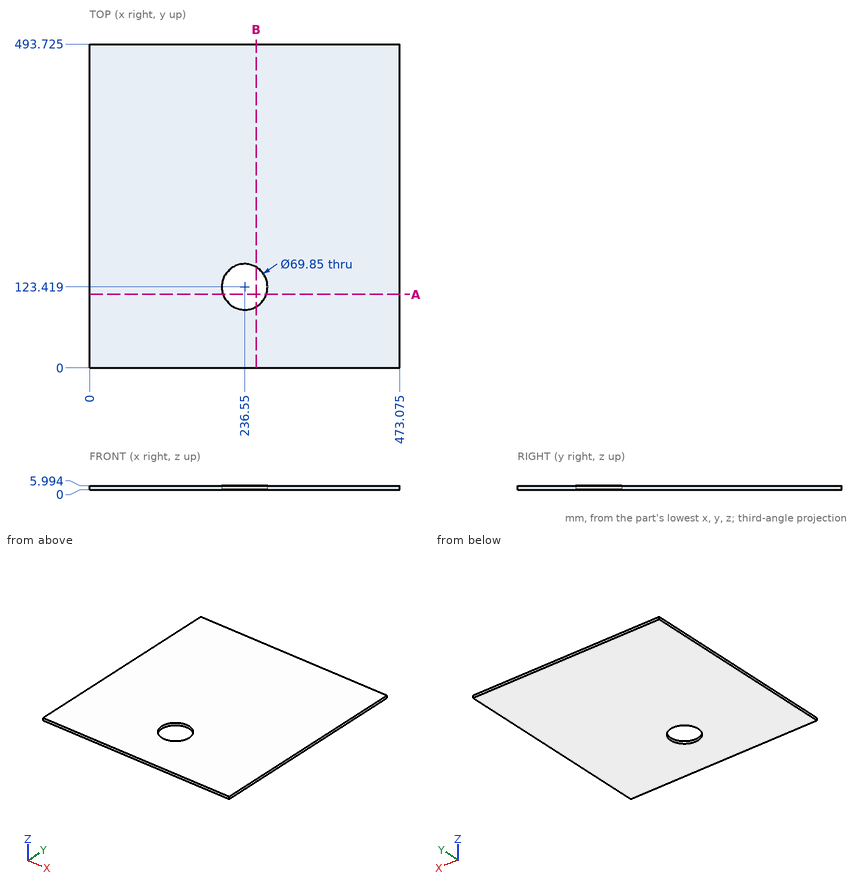
Could you check a few things on this drawing? It's one solid part, dimensions in mm from its lowest x, y, z. Coordinates: 2 decimals unless noted, no trailing zeros. Write each loop counter-clockwise with the first axis right and the second up, starting at its lowest first coordinate (ties: lowest second). Pieces come first, ordered by that corner, then holes.
Q1. Please list where these lines run through material, in increasing order: L1, parallel to X at y = 133.5, z = 4.2 (1 decimal); L2, parallel to Y at x = 240.5, z = 1.9 (1 decimal); L3, parallel to Y at x = 211, z = 4.6 (1 decimal).
Results found:
L1: x = 0 to 203.1, 270 to 473.1
L2: y = 0 to 88.7, 158.1 to 493.7
L3: y = 0 to 99.6, 147.2 to 493.7
Q2. Imagine slicing it at B-B, the plane x = 254. List the corners of the cut face in (y, z) for me (1 decimal), plus the area to 3 significant figures.
Results found:
outline: (0, 0) - (93.2, 0) - (93.2, 6) - (0, 6) - close; (153.7, 0) - (493.7, 0) - (493.7, 6) - (153.7, 6) - close
area: 2,600 mm2
Q3. Imagine slicing it at A-A, the plane y = 112. List the corners of the cut face in (x, z) for me (1 decimal).
Results found:
outline: (0, 0) - (203.5, 0) - (203.5, 6) - (0, 6) - close; (269.6, 0) - (473.1, 0) - (473.1, 6) - (269.6, 6) - close
